Geometry: final body of the model. Coordinates: model frame, mm. A direction names the side the tool comes from. Round coordinates to 2 decimals unless told otherwise and drop trailing zeros. Order: outer loops, then holes, each group sorted by start corner. A loop starts at its lowest first (then second) coordinate and runs counter-clockwise, first axis right, second up. Notation, with made-up numbers: M -31.5,42 L 2.5,42 A16 cw 2.5,59 Z; hole C -37.5,48 d4. An arc over 180 degrees is marked long. Return JSON: item names as keys, results as strings. Group by question number.
Q1. Cut plane B-B on x = 0. Output: boundary loops of the cut face in (y, z).
Q2. Ray query, probe 1 along Z at (x, y) = (0, 33); probe 2 along Z at (x, y) = (0, 96). Return the intervals inside material, ascending.
Q3. Contact query for flat-ended pins moving along their axis: pin 1 (1 mm diameter, centred on y = 53, z = 12.5, fed in from +X); pin 2 (12 mm diameter, centred on y = 84.5, z = 23, fed in from -X); pin 3 (12 mm diameter, centred on x = 16, y = 64, fed in from +Z). Output: stop coordinate, or through.
Q4. Cut plane C-C on y = 37. Output: boundary loops of the cut face in (x, z).
Q5. Access query for faces 4 (the face through (-26, 110.6, -11)), 5 (the face through (-3.788, 97.042, -28.852)). Directions: +Z, -Z, +X, -X, +Y, -Y. A direction counts if a zero-diameter tool reaches every point of the face in a straight line with its end or side. Return the directions, or none.
Q6. Mould query, pull axis Z, two halves, no side actions, for faces 1 (the face through (15.993, 75.952, -25.085)), 2 (the face through (-14.18, 0, 24.04)), 3 (the face through (-26.469, 54.526, -8.335)). Classes: released by +Z, released by -Z, zero draft, split by the parting line, or undercut.
Q7. Cut plane D-D on y = 74. Output: boundary loops of the cut face in (x, z).
Q8. Cut plane A-A on z = 0. Output: boundary loops of the cut face in (x, y).
Autodesk Inventor part; units mm, degrees
ref_plane "Work Plane1" through (0, 7.749, 0) normal (0, 1, 0) x (-1, 0, 0)
ref_plane "Work Plane2" through (0, 16.1, 0) normal (0, 1, 0) x (-1, 0, 0)
ref_plane "Work Plane3" through (0, 113.3, 0) normal (0, 1, 0) x (-1, 0, 0)
sketch "Sketch1" plane through (0, 0, 0) normal (0, 1, 0) x (-1, 0, 0)
  circle A0 centre (0, 0) radius 27.75
  circle A1 centre (0, 0) radius 32.25
  dimension "d0" = 55.5
  dimension "d1" = 64.5
extrude "Extrusion1" add sketch "Sketch1" along normal blind 110.6
ref_plane "Work Plane1" through (0, 7.749, 0) normal (0, 1, 0) x (-1, 0, 0)
ref_plane "Work Plane2" through (0, 16.1, 0) normal (0, 1, 0) x (-1, 0, 0)
ref_plane "Work Plane3" through (0, 113.3, 0) normal (0, 1, 0) x (-1, 0, 0)
sketch "Sketch17" plane through (0, 110.6, 0) normal (0, 1, 0) x (1, 0, 0)
  circle A0 centre (0, 0) radius 29.75
  circle A1 centre (0, 0) radius 32.25
  dimension "d109" = 59.5
extrude "Extrusion8" cut sketch "Sketch17" against normal blind 42
thread "Thread7"
sketch "Sketch18" plane through (0, 110.6, 0) normal (0, 1, 0) x (1, 0, 0)
  circle A0 centre (0, 0) radius 32.1723
  circle A1 centre (0, 0) radius 29.1
  dimension "d114" = 58.2
extrude "Extrusion9" cut sketch "Sketch18" against normal blind 27.5
properties part number "Vacuum Cylinder"
Result sheet:
{
 "1": {"outline": "M 0,-32.25 L 68.6,-32.25 L 68.6,-29.75 L 83.1,-29.75 L 83.1,-29.1 L 110.6,-29.1 L 110.6,-27.75 L 0,-27.75 Z; M 0,27.75 L 110.6,27.75 L 110.6,29.1 L 83.1,29.1 L 83.1,29.75 L 68.6,29.75 L 68.6,32.25 L 0,32.25 Z"},
 "2": {"probe 1": "z = -32.25 to -27.75, 27.75 to 32.25", "probe 2": "z = -29.1 to -27.75, 27.75 to 29.1"},
 "3": {"pin 1": "stops at x = 29.93", "pin 2": "stops at x = -24.3", "pin 3": "stops at z = 30.66"},
 "4": {"outline": "C 0,0 d64.5; hole C 0,0 d55.5"},
 "5": {"face 4": "+Z, -Z, +X, -X, +Y", "face 5": "+Y"},
 "6": {"face 1": "split by the parting line", "face 2": "zero draft", "face 3": "undercut"},
 "7": {"outline": "C 0,0 d59.5; hole C 0,0 d55.5"},
 "8": {"outline": "M -32.25,0 L -27.75,0 L -27.75,110.6 L -29.1,110.6 L -29.1,83.1 L -29.75,83.1 L -29.75,68.6 L -32.25,68.6 Z; M 27.75,0 L 32.25,0 L 32.25,68.6 L 29.75,68.6 L 29.75,83.1 L 29.1,83.1 L 29.1,110.6 L 27.75,110.6 Z"}
}
